Geometry check sheet. Reference: the model listing, model coordinates, mm. A direction names the side the tool comes from. Coordinates: 2 decimals unless noted, no trailing zeros. Order: outer loops, then holes, each group sorted by start corner. A loop starts at its lowest first (then second) coordinate and runs counter-clockwise, first axis right, second up. Notation, with made-up numbers: (35, 23.5) - (73, 23.5) arc R8 cw to (73, 29.5) - close; hole circle Ø8 at (15.5, 30.25). An arc over 180 degrees is marked (long way). One line per item, written item: value. Start each with the question number.
Autodesk Inventor part; units mm, degrees
ref_plane "YZ Plane" through (0, 0, 0) normal (1, 0, 0) x (0, 1, 0)
ref_plane "XZ Plane" through (0, 0, 0) normal (0, 1, 0) x (-1, 0, 0)
ref_plane "XY Plane" through (0, 0, 0) normal (0, 0, 1) x (1, 0, 0)
sketch "Esboço1" plane through (0, 0, 0) normal (0, 1, 0) x (-1, 0, 0)
  line L0 (-93, -3) -> (0, -3)
  line L1 (0, -25) -> (-58, -25)
  line L2 (-93, 0) -> (-93, -28)
  line L3 (-93, -28) -> (-83, -28)
  line L4 (-55, -28) -> (0, -28)
  line L5 (0, -28) -> (0, 0)
  line L6 (0, 0) -> (-93, 0)
  line L7 (-55, -28) -> (-55, -53)
  line L8 (-55, -53) -> (-93, -53)
  line L9 (-93, -53) -> (-93, -50)
  line L10 (-93, -50) -> (-58, -50)
  line L11 (-58, -50) -> (-58, -25)
  arc A0 (-83, -50) -> (-58, -25) centre (-83, -25) ccw
  arc A1 (-83, -28) -> (-80, -25) centre (-83, -25) ccw
  line L12 (-93, -25) -> (-80, -25)
  line L13 (0, 0) -> (3, 0)
  line L14 (3, 0) -> (3, -28)
  line L15 (3, -28) -> (0, -28)
  line L16 (-83, -28) -> (-83, -25)
  line L17 (-93, -50) -> (-93, -28)
  point P0 (-93, -14)
  point P1 (-93, -51.5)
  point P2 (-83, -28)
  dimension "d7" = 22
  dimension "d9" = 3
  dimension "d10" = 3
  dimension "d13" = 3
  dimension "d14" = 3
  dimension "d16" = 22
  dimension "d20" = 22
  dimension "d21" = 80
  dimension "d29" = 3
  dimension "d31" = 10
extrude "Extrusão1" add sketch "Esboço1" against normal blind 3
extrude "Extrusão2" add sketch "Esboço1" along normal blind 10 contours L2 L6 L5 L0 | L5 L13 L14 L15 | L12 L16 L3 L2 | L5 L4 L7 L8 L9 L10 L11 L1
equation "\"d9\" = mdf"
equation "\"d10\" = mdf"
equation "\"d13\" = mdf"
equation "\"d14\" = mdf"
equation "\"mdf\" = 3"
equation "\"margem\" = 1"
properties part number "Trilho 5 min"
Q1. Cross-section at A-A, the plane y = 7.25. Enter the section's corners in (x, z), and give its area (3 significant figures).
Q2. Release check for a two-part mould opening along X. For faces 4 (the flat face through (83, 5, -27)), 5 (the flat face through (0, 5, -14)), 6 (the flat face through (76, 5, -50)) record: released by +X, released by -X, zero draft, split by the parting line, or undercut.
Q3. Cross-section at B-B, the plane x = 60. Enter the section's corners in (y, z).
Q4. Cross-section at D-D, the plane x = 37. Enter the section's corners in (y, z).
Q5. Material ranges on probe 1 along Z at (x, y) = (88, 1.25); probe 2 along Z at (x, y) = (35.5, 3.75); probe 3 along Z at (x, y) = (61.5, 9), recorded low to high.
Q6. Set-up check for faces 1 (the flat face through (55, 4, -40)), 2 (the flat face through (29, 5, -25)), 3 (the flat face through (93, -1, -20)): record each of +Z, -Z, +X, -X, +Y, -Y from which the full face is reachable in a straight line by a thin tool's end or side.
Q7. Cross-section at C-C, the plane z = -23.5. Enter the section's corners in (x, y).
Q8. Gauge pin test, flat ends, axial feed: P1, Ø8, axis at x = 79, z = -33, coming from the +Y side; P2, Ø4, axis at y = 5.5, z = -32, coming from the +X side; P3, Ø3, axis at y = 6.5, z = -14.5, coming from the +X side. Record the tip position at first contact, or that the pin passes through.
Check result:
1. outline: (-3, -28) - (55, -28) - (55, -53) - (93, -53) - (93, -50) - (58, -50) - (58, -25) - (0, -25) - (0, -3) - (93, -3) - (93, 0) - (-3, 0) - close; (83, -28) - (93, -28) - (93, -25) - (83, -25) - close
1. area: 747 mm2
2. face 4: undercut
2. face 5: released by +X
2. face 6: zero draft
3. outline: (-3, -53) - (10, -53) - (10, -50) - (0, -50) - (0, -3) - (10, -3) - (10, 0) - (-3, 0) - close
4. outline: (-3, -28) - (10, -28) - (10, -25) - (0, -25) - (0, -3) - (10, -3) - (10, 0) - (-3, 0) - close
5. probe 1: z = -53 to -50, -28 to -25, -3 to 0
5. probe 2: z = -28 to -25, -3 to 0
5. probe 3: z = -53 to -50, -3 to 0
6. face 1: -Z, -X, +Y, -Y
6. face 2: +X, +Y
6. face 3: +Z, -Z, +X, +Y, -Y
7. outline: (-3, -3) - (93, -3) - (93, 0) - (0, 0) - (0, 10) - (-3, 10) - close
8. P1: stops at y = 0
8. P2: stops at x = 58
8. P3: stops at x = 0
